Verification items for this drawing (mm, ordinates from the low corner). A direction names the side the tool comes from. Give positions to 0.01 mm unless a question says otherwise; leave off trailing zeros. Loops run counter-clockwise (first coordinate to the right, second up) from the corner with the lowest first, then second, coordinate; pieces in that order, holes last. Notation, with made-up numbers: (75.25, -24.75) -> (101.25, -24.75) arc R25 cw to (101.25, -0.75) -> close; hole circle Ø9 at (18, 84.5). An arc over 180 degrees is marked (long way). Write each question's results on one line, items separated by ' | '. Start each with the question number.
Item 1: Scan lines: line 1 along X through (y, z) = (1.55, 36); line 2 along Y through (x, z) = (32.5, 22); line 3 along Y through (x, z) = (10.5, 21). Record each from-to range of solid material in increasing order.
Item 2: Cross-section at D-D on y = 9. Enter the section's corners in (x, z), then the cut area to 3 significant figures.
Item 3: Cross-section at B-B on z = 36. Enter the section's corners in (x, y).
Item 4: Cross-section at C-C on x = 19. Enter the section's corners in (y, z), then the cut area to 3 significant figures.
Item 5: Access from +Z, -Z, +X, -X, +Y, -Y to the whole of each face (thin tool, end or side, straight path). Record for the marked faces 1 and 2.
Item 6: Gauge pin test, flat ends, axial feed: pin 1 Ø5 at (y, z) = (14, 18) entering from +X; pin 2 Ø1 at (y, z) = (19, 25) entering from -X; pin 3 Ø1 at (x, y) = (23.5, 20) entering from +Z. Record the tip position at first contact, or that the pin passes through.
Item 7: Cross-section at A-A on x = 2. Enter the section's corners in (y, z).
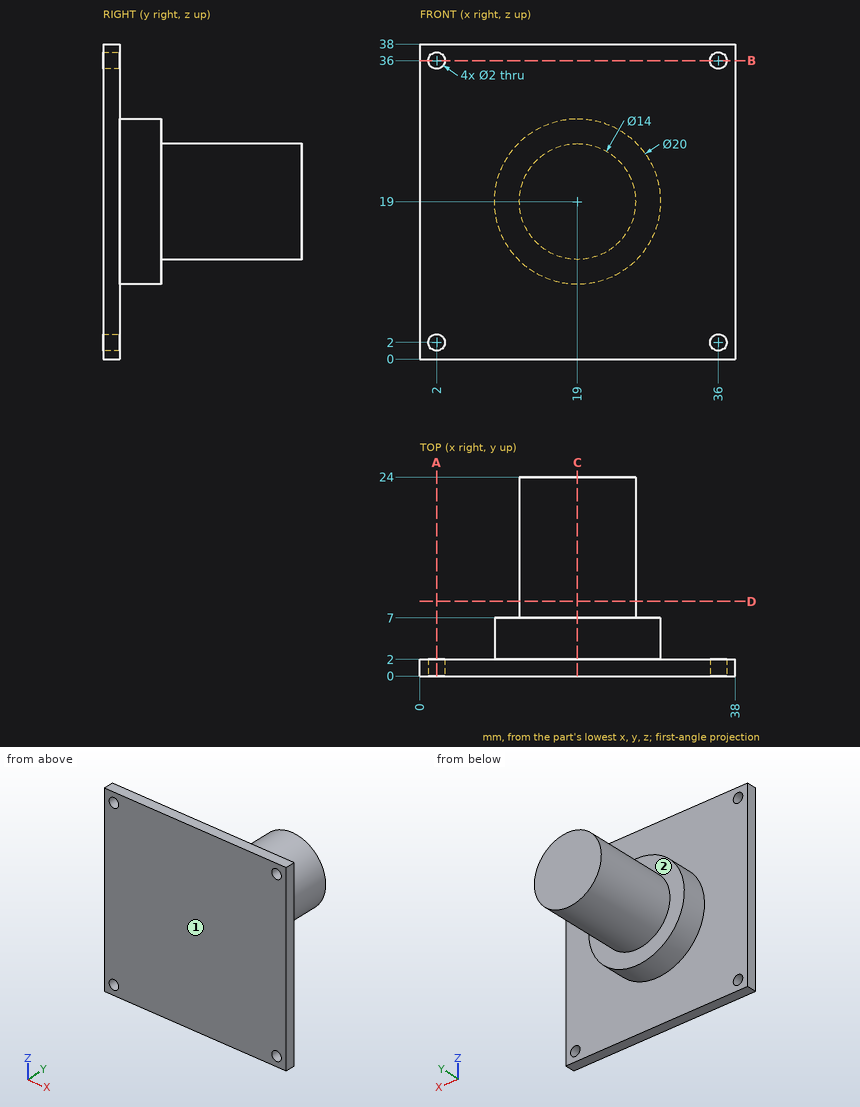
Answer sheet:
1) line 1: x = 0 to 1, 3 to 35, 37 to 38 | line 2: y = 0 to 2 | line 3: y = 0 to 7
2) outline: circle Ø14 at (19, 19) | area: 154 mm²
3) outline: (0, 0) -> (1, 0) -> (1, 2) -> (0, 2) -> close; (3, 0) -> (35, 0) -> (35, 2) -> (3, 2) -> close; (37, 0) -> (38, 0) -> (38, 2) -> (37, 2) -> close
4) outline: (0, 0) -> (2, 0) -> (2, 9) -> (7, 9) -> (7, 12) -> (24, 12) -> (24, 26) -> (7, 26) -> (7, 29) -> (2, 29) -> (2, 38) -> (0, 38) -> close | area: 414 mm²
5) face 1: +Z, -Z, +X, -X, -Y | face 2: +Y
6) pin 1: stops at x = 26 | pin 2: stops at x = 14.67 | pin 3: stops at z = 24.74
7) outline: (0, 0) -> (2, 0) -> (2, 1) -> (0, 1) -> close; (0, 3) -> (2, 3) -> (2, 35) -> (0, 35) -> close; (0, 37) -> (2, 37) -> (2, 38) -> (0, 38) -> close
